from build123d import *

# Parameters (mm, degrees)
PAD_DEPTH    = 17.7
POCKET_DEPTH = 6.1
SKETCH004_R  = 5.5
PAD001_DEPTH = 9.65
SKETCH005_R  = 5.5
PAD002_DEPTH = 9.65


with BuildPart() as obj1:
    # Sketch002 → Loft section 0
    with BuildSketch(Plane.XY):
        with BuildLine():
            Line((32.6, -42.200036), (32.6, -60))
            Line((32.6, -60), (19, -60))
            Line((19, -60), (19, -42.200036))
            ThreePointArc((32.6, -42.200036), (25.8, -35.4), (19, -42.200036))
        make_face()
    # Sketch003 → Loft section 1
    with BuildSketch(Plane.XY.offset(12.5)):
        with BuildLine():
            Line((34.8, -42.4), (34.8, -61))
            Line((34.8, -61), (16.8, -61))
            Line((16.8, -61), (16.8, -42.4))
            ThreePointArc((34.8, -42.4), (25.8, -33.4), (16.8, -42.4))
        make_face()
    loft(ruled=True)


with BuildPart() as base:
    # Sketch → Pad (new body)
    with BuildSketch(Plane.XY):
        with BuildLine():
            Line((0, 0), (51.1, 0))
            Line((51.1, 0), (51.1, -53))
            ThreePointArc((45.1, -59), (49.342641, -57.242641), (51.1, -53))
            Line((45.1, -59), (6, -59))
            ThreePointArc((0, -53), (1.757359, -57.242641), (6, -59))
            Line((0, -53), (0, 0))
        make_face()
    extrude(amount=PAD_DEPTH)

    # Sketch001 → Pocket (cut)
    with BuildSketch(Plane.XY.offset(17.7)):
        with BuildLine():
            Line((39.35, -41.3), (39.35, -59))
            Line((11.75, -59), (39.35, -59))
            Line((11.75, -59), (11.75, -41.3))
            ThreePointArc((39.35, -41.3), (25.55, -27.5), (11.75, -41.3))
        make_face()
    extrude(amount=-POCKET_DEPTH, mode=Mode.SUBTRACT)

    # Cut: cut obj1
    add(obj1.part, mode=Mode.SUBTRACT)


with BuildPart() as obj2:
    # Sketch004 → Pad001 (new body)
    with BuildSketch(Plane.YZ):
        with BuildLine():
            Line((0, 39.9), (0, 0))
            Line((0, 0), (-25.5, 0))
            Line((-25.5, 0), (-25.5, 39.9))
            ThreePointArc((0, 39.9), (-12.75, 52.65), (-25.5, 39.9))
        make_face()
        with Locations((-12.75, 39.9)):
            Circle(SKETCH004_R, mode=Mode.SUBTRACT)
    extrude(amount=PAD001_DEPTH)


with BuildPart() as obj3:
    # Sketch005 → Pad002 (new body)
    with BuildSketch(Plane.YZ.offset(51.1)):
        with BuildLine():
            Line((0, 39.9), (0, 0))
            Line((0, 0), (-25.5, 0))
            Line((-25.5, 0), (-25.5, 39.9))
            ThreePointArc((0, 39.9), (-12.75, 52.65), (-25.5, 39.9))
        make_face()
        with Locations((-12.75, 39.9)):
            Circle(SKETCH005_R, mode=Mode.SUBTRACT)
    extrude(amount=-PAD002_DEPTH)

    # Fusion: union obj2
    add(obj2.part)

    # Fusion001: union Base
    add(base.part)


solid = obj3.part
Can you work these out from the model? Positions are in its coordinate system, mm. A direction names the side the tool comes from. Give positions to 0.01 mm unless a question says otherwise; leave off trailing zeros. Loops run counter-clockwise (first coordinate to the right, second up) from the corner with the lowest first, then second, coordinate; pieces in that order, holes last. Notation, with made-up numbers: (29.25, -19) -> (72.25, -19) arc R14 ccw to (72.25, 1) -> close; hole circle Ø9 at (64.25, -16.75). An arc over 180 degrees is marked (long way). Use one line per item in the form item = value.
1) If we section it at D-D (z = 44.5): Please give me the cut outline in (x, y).
Answers:
outline = (0, -24.64) -> (9.65, -24.64) -> (9.65, -15.76) -> (0, -15.76) -> close; (0, -9.74) -> (9.65, -9.74) -> (9.65, -0.86) -> (0, -0.86) -> close; (41.45, -24.64) -> (51.1, -24.64) -> (51.1, -15.76) -> (41.45, -15.76) -> close; (41.45, -9.74) -> (51.1, -9.74) -> (51.1, -0.86) -> (41.45, -0.86) -> close
2) I need wall thicknesses on line 1 along X through (y, z) = (-17, 23.5); line 2 along Z through (x, y) = (5, -12.75); line 3 along Z through (x, y) = (31, -11.5). Which ranges of each line are inside material? Lowest first, please.
Answers:
line_1 = 0 to 9.65, 41.45 to 51.1
line_2 = 0 to 34.4, 45.4 to 52.65
line_3 = 0 to 17.7
3) Will these pins go through, and if not, where does the flat tip stop? pin 1 (3 mm diameter, centred on x = 47, z = 24, fed in from -Y); pin 2 (4 mm diameter, centred on x = 38, y = -50, fed in from +Z); pin 3 (1.5 mm diameter, centred on x = 26, z = 12, fed in from -Y).
Answers:
pin_1 = -25.5
pin_2 = 17.7
pin_3 = -33.6
4) We'd pull the mould along X, two halves only. Please class faces 1 (the face through (0, -20, 21)), 2 (the face through (4.757, -9.793, 44.538)), 3 (the face through (26, -23, 17.7)), 4 (the face through (16.5, -43, 11.6)): released by +X, released by -X, zero draft, split by the parting line, or undercut.
Answers:
face_1 = released by -X
face_2 = zero draft
face_3 = undercut
face_4 = undercut
5) If we section it at B-B (x = 48): Please give me the cut outline in (y, z), plus the area to 3 significant figures.
Answers:
outline = (-58.25, 0) -> (0, 0) -> (0, 39.9) arc R12.75 ccw to (-25.5, 39.9) -> (-25.5, 17.7) -> (-58.25, 17.7) -> close; hole circle Ø11 at (-12.75, 39.9)
area = 1,760 mm²
6) If we section it at A-A (z = 18.5): Please give me the cut outline in (x, y).
Answers:
outline = (0, -25.5) -> (9.65, -25.5) -> (9.65, 0) -> (0, 0) -> close; (41.45, -25.5) -> (51.1, -25.5) -> (51.1, 0) -> (41.45, 0) -> close
7) If we section it at C-C (y = -13.5): Please give me the cut outline in (x, z), plus the area to 3 significant figures.
Answers:
outline = (0, 0) -> (51.1, 0) -> (51.1, 34.45) -> (41.45, 34.45) -> (41.45, 17.7) -> (9.65, 17.7) -> (9.65, 34.45) -> (0, 34.45) -> close; (0, 45.35) -> (9.65, 45.35) -> (9.65, 52.63) -> (0, 52.63) -> close; (41.45, 45.35) -> (51.1, 45.35) -> (51.1, 52.63) -> (41.45, 52.63) -> close
area = 1,370 mm²
8) For faces 5 (the face through (46, -25.5, 29)), 6 (the face through (25.853, -27.503, 14.693)), 7 (the face through (9.65, -13, 32)), which set-ups out of +Z, -Z, +X, -X, +Y, -Y let a thin tool reach every point of the face, with its end or its side?
Answers:
face_5 = +Z, +X, -X, -Y
face_6 = +Z, -Y
face_7 = +Z, +Y, -Y
